Check sheet for the modelled part. Datum: model origin and axes. Units: mm. A direction names the side the tool comes from. Give positions to 0.01 mm unless a question says otherwise; leave off trailing zeros. Write each loop counter-clockwise with the first axis right and the second up, starting at its lowest first coordinate (ties: lowest second). Pieces come first, ordered by that corner, then holes. Notation, with made-up numbers: (76, -6.5) -> (134, -6.5) arc R37 cw to (134, 29.5) -> close; hole circle Ø3 at (-16.5, 2). An arc over 180 degrees is marked (long way). Use a Markdown table: item, result. Add a question column.
1. Cross-section at B-B (y = 20.5). Enter the section's corners in (x, z), then the cut area to 3 significant figures.
2. Set-up check for faces 4 (the flat face through (-73.252, 54.942, 7.028)), 5 (the flat face through (-92.152, 48.562, 5.76)), 6 (the flat face through (-80.59, -16.46, 5.76)): record each of +Z, -Z, +X, -X, +Y, -Y from which the full face is reachable in a straight line by a thin tool's end or side.
3. Release check for a two-part mould opening along X. For faces 1 (the flat face through (-100.553, 43.147, 7.028)), 2 (the flat face through (-99, 16, 0)), 3 (the flat face through (-52.53, 38.21, 5.76)) record: released by +X, released by -X, zero draft, split by the parting line, or undercut.
4. Cross-section at C-C (x = -52.5). Enter the section's corners in (y, z), then the cut area to 3 significant figures.
5. Scan lines: probe 1 along Z at (x, y) = (-110, 20.5); probe 2 along Y at (x, z) = (-133.5, 6.25); probe 3 along Y at (x, z) = (-101, 5.75). Record each from-to range of solid material in increasing order. Write a range as [from, to].
6. Cross-section at A-A (z = 7.25). Enter the section's corners in (x, y), then the cut area to 3 significant figures.
7. Gauge pin test, flat ends, axial feed: P1, Ø5, axis at y = -12, z = 8, coming from the -X side (3 decimals); P2, Ø10, axis at x = -92.5, y = -5.5, coming from the +Z side; P3, Ø2, axis at y = 18.5, z = 3.5, coming from the +X side. Record the tip position at first contact, or that the pin passes through.
from build123d import *

# Parameters (mm, degrees)
F1_DEPTH = 11.684
F2_DEPTH = 25
F3_DEPTH = 13
F4_T     = -2.5


with BuildPart() as f1:
    # F0 (on Top) → F1 (new body)
    with BuildSketch(Plane.XY):
        with BuildLine():
            Line((-101.0389998555, 31.3125476241), (-114.6383360028, 39.1371101141))
            ThreePointArc((-114.6383360028, 39.1371101141), (-148.8700631478, 25.8791054822), (-122.8343620896, 0))
            Line((-122.8343620896, 0), (-47.8479606974, 16.1763411877))
            Line((-47.8479606974, 16.1763411877), (-57.3485940695, 60.8779378235))
            Line((-57.3485940695, 60.8779378235), (-89.3066003919, 54.0857575834))
            Line((-89.3066003919, 54.0857575834), (-101.0389998555, 31.3125476241))
        make_face()
    extrude(amount=F1_DEPTH)

    # F2 (add): a face of the model
    f2_faces = [f1.faces().sort_by_distance(p)[0] for p in [
        (-85.3411613935, 8.0881705939, 5.842),
    ]]
    extrude(f2_faces, amount=F2_DEPTH)

    # F3 (add): a face of the model
    f3_faces = [f1.faces().sort_by_distance(p)[0] for p in [
        (-107.8386679292, 35.2248288691, 5.842),
    ]]
    extrude(f3_faces, amount=F3_DEPTH)

    # F4
    f4_openings = [f1.faces().sort_by_distance(p)[0] for p in [
        (-92.967353, 17.456515, 11.684),
    ]]
    offset(amount=F4_T, openings=f4_openings, kind=Kind.INTERSECTION)


solid = f1.part
Worked answers:
| question | item | result |
|---|---|---|
| 1 | outline | (-149.32, 0) -> (-48.77, 0) -> (-48.77, 11.68) -> (-51.32, 11.68) -> (-51.32, 2.5) -> (-146.81, 2.5) -> (-146.81, 11.68) -> (-149.32, 11.68) -> close |
| 1 | area | 298 mm² |
| 2 | face 4 | +Z |
| 2 | face 5 | +Z, -Z, +Y |
| 2 | face 6 | +Z, -Z, +X, -Y |
| 3 | face 1 | undercut |
| 3 | face 2 | zero draft |
| 3 | face 3 | released by +X |
| 4 | outline | (-10.4, 0) -> (38.06, 0) -> (38.06, 11.68) -> (26.04, 11.68) -> (26.04, 2.5) -> (-7.84, 2.5) -> (-7.84, 11.68) -> (-10.4, 11.68) -> close |
| 4 | area | 255 mm² |
| 5 | probe 1 | z = [0, 2.5] |
| 5 | probe 2 | y = [0.36, 2.98], [39.81, 42.43] |
| 5 | probe 3 | y = [-20.86, -18.31], [43.4, 46.29] |
| 6 | outline | (-122.83, 0) -> (-117.56, -24.44) -> (-42.58, -8.26) -> (-47.85, 16.18) -> (-57.35, 60.88) -> (-89.31, 54.09) -> (-95.08, 42.88) -> (-108.16, 50.41) -> (-114.64, 39.14) arc R21.89 ccw (long way) to start; hole (-120.95, 3.13) -> (-115.65, -21.47) -> (-45.55, -6.34) -> (-50.29, 15.65) -> (-59.27, 57.91) -> (-87.63, 51.89) -> (-94.06, 39.41) -> (-107.23, 46.99) -> (-113.96, 35.31) arc R19.39 ccw (long way) to start |
| 6 | area | 812 mm² |
| 7 | P1 | stops at x = -120.785 |
| 7 | P2 | stops at z = 2.5 |
| 7 | P3 | stops at x = -48.13 |
